```python
from build123d import *

# Parameters (mm, degrees)
BOSS_EXTRUDE1_DEPTH = 15
SKETCH2_W           = 32.3
SKETCH2_H           = 2.5
BOSS_EXTRUDE2_DEPTH = 23.5
SKETCH3_W           = 5
SKETCH3_H           = 6.2
CUT_EXTRUDE1_DEPTH  = 12.5
CUT_EXTRUDE2_REACH  = 28
SKETCH4_R           = 3.9
SKETCH5_R           = 1.2
CUT_EXTRUDE3_DEPTH  = 2.5
CUT_EXTRUDE4_REACH  = 39.3
SKETCH6_R           = 1.55
FILLET2_R           = 2
SKETCH7_W           = 8
SKETCH7_H           = 8
SKETCH7_R           = 1.55
CUT_EXTRUDE5_DEPTH  = 1.5
CUT_EXTRUDE6_REACH  = 4.5
SKETCH8_RX          = 9.634046057
SKETCH8_RY          = 6.312870092
SKETCH8_W           = 10.5
SKETCH8_H           = 3.175


with BuildPart() as part:
    # Sketch1 → Boss-Extrude1 (new body)
    with BuildSketch(Plane(origin=(0, 0, 0), x_dir=(1, 0, 0), z_dir=(0, 1, 0))):
        Polygon((0, 29.994099724), (-26, 29.994099724), (-26, -7.305900276), (0, -7.305900276), (0, -0.005900276), (-2.5, -0.005900276), (-2.5, -4.805900276), (-23.5, -4.805900276), (-23.5, 27.494099724), (-2.5, 27.494099724), (-2.5, 22.694099724), (0, 22.694099724), align=None)
    extrude(amount=BOSS_EXTRUDE1_DEPTH)

    # Sketch2 → Boss-Extrude2 (add, through all)
    with BuildSketch(Plane(origin=(-23.5, 0, 0), x_dir=(0, 0, -1), z_dir=(1, 0, 0))):
        with Locations((11.344099724, 1.25)):
            Rectangle(SKETCH2_W, SKETCH2_H)
    extrude(amount=BOSS_EXTRUDE2_DEPTH)

    # Sketch3 → Cut-Extrude1 (cut)
    with BuildSketch(Plane(origin=(0, 0, -29.994099724), x_dir=(-1, 0, 0), z_dir=(0, 0, -1))):
        with Locations((16.375, 8.6)):
            Rectangle(SKETCH3_W, SKETCH3_H)
    extrude(amount=-CUT_EXTRUDE1_DEPTH, mode=Mode.SUBTRACT)

    # Sketch4 → Cut-Extrude2 (cut, up to next)
    with BuildSketch(Plane.ZY.offset(26), mode=Mode.PRIVATE) as cut_extrude2_sk1:
        with Locations((-16.544099724, 8.6)):
            Circle(SKETCH4_R)
    cut_extrude2_tool1 = extrude(cut_extrude2_sk1.sketch, amount=-CUT_EXTRUDE2_REACH, mode=Mode.PRIVATE) & part.part
    add(cut_extrude2_tool1.solids().sort_by_distance((-26, 8.6, -16.5441))[0], mode=Mode.SUBTRACT)

    # Sketch5 → Cut-Extrude3 (cut)
    with BuildSketch(Plane(origin=(0, 0, 0), x_dir=(0, 0, -1), z_dir=(1, 0, 0))):
        with Locations((-2.555900276, 8.6)):
            Circle(SKETCH5_R)
    cut_extrude3 = extrude(amount=-CUT_EXTRUDE3_DEPTH, mode=Mode.SUBTRACT)

    # Mirror1: Cut-Extrude3 across plane
    add(cut_extrude3.mirror(Plane.XY.offset(-11.344099724)), mode=Mode.SUBTRACT)

    # Sketch6 → Cut-Extrude4 (cut, up to next)
    with BuildSketch(Plane.XY.offset(7.305900276), mode=Mode.PRIVATE) as cut_extrude4_sk1:
        with Locations((-13, 8.75)):
            Circle(SKETCH6_R)
    cut_extrude4_tool1 = extrude(cut_extrude4_sk1.sketch, amount=-CUT_EXTRUDE4_REACH, mode=Mode.PRIVATE) & part.part
    add(cut_extrude4_tool1.solids().sort_by_distance((-13, 8.75, 7.3059))[0], mode=Mode.SUBTRACT)

    # Fillet2
    fillet2_edges = [part.edges().sort_by_distance(p)[0] for p in [
        (0, 0, -11.344099724),
        (-13, 0, 7.305900276),
        (-26, 0, -11.344099724),
        (-13, 0, -29.994099724),
        (0, 7.5, 7.305900276),
        (-26, 7.5, 7.305900276),
        (-26, 7.5, -29.994099724),
        (0, 7.5, -29.994099724),
    ]]
    fillet(fillet2_edges, radius=FILLET2_R)

    # Sketch7 → Cut-Extrude5 (cut)
    with BuildSketch(Plane.XY.offset(7.305900276)):
        with Locations((-13, 8.75)):
            Rectangle(SKETCH7_W, SKETCH7_H)
        with Locations((-13, 8.75)):
            Circle(SKETCH7_R, mode=Mode.SUBTRACT)
    extrude(amount=-CUT_EXTRUDE5_DEPTH, mode=Mode.SUBTRACT)

    # Sketch8 → Cut-Extrude6 (cut, up to next)
    with BuildSketch(Plane(origin=(0, 2.5, 0), x_dir=(1, 0, 0), z_dir=(0, 1, 0)), mode=Mode.PRIVATE) as cut_extrude6_sk1:
        with Locations(Location((-13, 11.344099724), (0, 0, 90))):
            Ellipse(SKETCH8_RX, SKETCH8_RY)
    cut_extrude6_tool1 = extrude(cut_extrude6_sk1.sketch, amount=-CUT_EXTRUDE6_REACH, mode=Mode.PRIVATE) & part.part
    add(cut_extrude6_tool1.solids().sort_by_distance((-13, 2.5, -11.3441))[0], mode=Mode.SUBTRACT)
    # Sketch8 → Cut-Extrude6 (cut, up to next)
    with BuildSketch(Plane(origin=(0, 2.5, 0), x_dir=(1, 0, 0), z_dir=(0, 1, 0)), mode=Mode.PRIVATE) as cut_extrude6_sk2:
        with Locations((-13, -2.231384095)):
            Rectangle(SKETCH8_W, SKETCH8_H)
    cut_extrude6_tool2 = extrude(cut_extrude6_sk2.sketch, amount=-CUT_EXTRUDE6_REACH, mode=Mode.PRIVATE) & part.part
    add(cut_extrude6_tool2.solids().sort_by_distance((-13, 2.5, 2.231384))[0], mode=Mode.SUBTRACT)
    # Sketch8 → Cut-Extrude6 (cut, up to next)
    with BuildSketch(Plane(origin=(0, 2.5, 0), x_dir=(1, 0, 0), z_dir=(0, 1, 0)), mode=Mode.PRIVATE) as cut_extrude6_sk3:
        with Locations((-13, 24.919583542)):
            Rectangle(SKETCH8_W, SKETCH8_H)
    cut_extrude6_tool3 = extrude(cut_extrude6_sk3.sketch, amount=-CUT_EXTRUDE6_REACH, mode=Mode.PRIVATE) & part.part
    add(cut_extrude6_tool3.solids().sort_by_distance((-13, 2.5, -24.919584))[0], mode=Mode.SUBTRACT)


solid = part.part
```
Can you work these out from the model? Positions are in its coordinate system, mm. A direction names the side the tool comes from. Coordinates: 2 decimals unless noted, no trailing zeros. Write each loop counter-clockwise with the first axis right and the second up, starting at its lowest first coordinate (ties: lowest second). Pieces come first, ordered by that corner, then holes. Notation, with made-up numbers: (-39.5, -7) - (-14.5, -7) arc R19 ccw to (-14.5, 4) - close; hole circle Ø11 at (3, 42). An arc over 180 degrees is marked (long way). Return JSON: item names as keys, results as strings.
Q1. Thinking about a two-plate mould opening in X: for faces 1 (the flat face through (-13, 1, 3.819)), 2 (the cylindrical face through (-0.57, 8.59, -29.39)), 3 (the flat face through (-13, 4, 7.306)), which applies, +X half, -X half, draft (parallel to the pull), parting line (faces both ways), or undercut?
Computed values:
{"face 1": "undercut", "face 2": "+X half", "face 3": "draft"}
Q2. I'm going to push flat-ended pins straight in: pin 1 Ø1.2 at (y, z) = (9, 6.5) entering from -X; pin 2 Ø8 at (x, z) = (-15.5, -26) entering from +Y; pin 3 Ø1.2 at (y, z) = (1, 1.5) entering from -X; pin 4 Ø4 at (y, z) = (10, -16) entering from +X. Where does each tip first touch, or does it pass through?
Computed values:
{"pin 1": "stops at x = -25.91", "pin 2": "stops at y = 15", "pin 3": "stops at x = -25.96", "pin 4": "passes through"}
Q3. If we section it at A-A (x = -4.75): Please give me the cut outline in (y, z).
Computed values:
{"outline": "(0, -27.99) arc R2 ccw to (2, -29.99) - (15, -29.99) - (15, -27.49) - (2.5, -27.49) - (2.5, 4.81) - (15, 4.81) - (15, 7.31) - (2, 7.31) arc R2 ccw to (0, 5.31) - close"}
Q4. If we section it at C-C (y = 6.5): Please give me the cut outline in (x, z) (3 decimals).
Computed values:
{"outline": "(-26, -27.994) arc R2 ccw to (-24, -29.994) - (-18.875, -29.994) - (-18.875, -27.494) - (-23.5, -27.494) - (-23.5, -19.83) - (-26, -19.83) - close; (-26, -13.258) - (-23.5, -13.258) - (-23.5, 4.806) - (-2.5, 4.806) - (-2.5, 0.006) - (0, 0.006) - (0, 5.306) arc R2 ccw to (-2, 7.306) - (-9, 7.306) - (-9, 5.806) - (-17, 5.806) - (-17, 7.306) - (-24, 7.306) arc R2 ccw to (-26, 5.306) - close; (-13.875, -29.994) - (-2, -29.994) arc R2 ccw to (0, -27.994) - (0, -22.694) - (-2.5, -22.694) - (-2.5, -27.494) - (-13.875, -27.494) - close"}
Q5. If we section it at D-D (x = -13): Count the separate pieces of the cut face and the enclosed holes in it, then the cut area to 3 significant figures.
Computed values:
{"separate pieces": "5", "enclosed holes": "0", "area": "74.9 mm2"}
Q6. Please list where these lines run through material, in increasing order: L1, parallel to Z at x = -13.5, y = 13; L2, parallel to Z at x = -9.25, y = 8; L3, parallel to Z at x = -8, y = 2.25. Write a range as from..to.
Computed values:
{"L1": "z = -29.99..-27.49, 4.81..7.31", "L2": "z = -29.99..-27.49, 4.81..5.81", "L3": "z = -29.99..-26.51, -23.33..-17.23, -5.46..0.64, 3.82..7.31"}
Q7. On a 3-axis mill with a long thin cutter (end or side, diameter ignored), from which of +Z, -Z, +X, -X, +Y, -Y can I reach the whole of each face in a straight line? I mean faces 4 (the flat face through (-23.5, 9, -11)), 5 (the flat face through (-13, 4.75, 7)), 6 (the cylindrical face through (-1.23, 8.96, -24.1)). Say none if no direction works.
Computed values:
{"face 4": "+Y", "face 5": "+Z", "face 6": "+X"}
Q8. If we section it at B-B (z = 3): Please give me the cut outline in (x, y).
Computed values:
{"outline": "(-26, 2) arc R2 ccw to (-24, 0) - (-18.25, 0) - (-18.25, 2.5) - (-23.5, 2.5) - (-23.5, 15) - (-26, 15) - close; (-7.75, 0) - (-2, 0) arc R2 ccw to (0, 2) - (0, 7.49) - (-2.5, 7.49) - (-2.5, 2.5) - (-7.75, 2.5) - close; (-2.5, 9.71) - (0, 9.71) - (0, 15) - (-2.5, 15) - close"}
